from build123d import *

# Parameters (mm, degrees)
BOSS_EXTRUDE1_DEPTH      = 40
BOSS_EXTRUDE2_DEPTH      = 10
BOSS_EXTRUDE2_DEPTH_BACK = 50
SKETCH3_R                = 55


with BuildPart() as part:
    # Sketch2 → Boss-Extrude1 (new body)
    with BuildSketch(Plane(origin=(0, 0, 0), x_dir=(1, 0, 0), z_dir=(0, 1, 0))):
        Polygon((-545, 0), (545, 0), (614.776428685, 27.5), (614.776428685, -82.5), (545, -55), (-545, -55), (-614.776428685, -82.5), (-614.776428685, 27.5), align=None)
    extrude(amount=BOSS_EXTRUDE1_DEPTH)

    # Sketch3 → Boss-Extrude2 (add, two sides: drawn at the far end of the back side and taken through both)
    with BuildSketch(Plane(origin=(0, 40, 0), x_dir=(1, 0, 0), z_dir=(0, 1, 0)).offset(-BOSS_EXTRUDE2_DEPTH_BACK)):
        with Locations(Location((-614.776428685, -27.5, 0), (0, 0, 270))):
            Circle(SKETCH3_R)
        with Locations(Location((614.776428685, -27.5, 0), (0, 0, 270))):
            Circle(SKETCH3_R)
    extrude(amount=BOSS_EXTRUDE2_DEPTH + BOSS_EXTRUDE2_DEPTH_BACK)


solid = part.part
Input: part model. Units: mm. Frame: model coordinates. A direction names the side the tool comes from. Coordinates: 2 decimals unless noted, no trailing zeros. Loops run counter-clockwise (first coordinate to the right, second up) from the corner with the lowest first, then second, coordinate; pieces in that order, holes last.
(1) Section B-B on y = 17.5. Return the cut outline in (x, z).
(2) Section A-A on z = 27.5. Return the cut outline in (x, y).
(3) Material intervals for probe 1 along Y at (x, z) = (248.5, 14); probe 2 along Z at (x, y) = (-511, 22.5); probe 3 along X at (y, z) = (-1.5, -23), sorted ascending.
(4) First-contact query: pin 1 Ø1.5 at (x, z) = (-123.5, 18.5) entering from -Y; pin 2 Ø12 at (x, y) = (-278.5, 36.5) entering from -Z; pin 3 Ø1.5 at (y, z) = (13.5, 68) entering from -X. Flat tips, straight axial feed; report the tip coordinate or a pass-through.
(5) Section C-C on x = -224. Return the cut outline in (y, z).
(6) Pull-direction query (X, two-part tool) for faces 1 (the face through (669.31, 19.58, 20.34)), 2 (the face through (616, 50, 27)), 3 (the face through (-561.352, 19.72, -6.445)); classes: released by +X, released by -X, zero draft, split by the parting line, or undercut.
(7) Set-up query: faces 4 (the face through (-8, 20, 0)), 5 (the face through (-614, 50, 27)), 6 (the face through (-560.9, 19.72, 61.267)). Return all of +Z, -Z, +X, -X, +Y, -Y with unobstructed straight access to the full face (end or side cutting, diameter ignored); none if empty.
Data:
1. outline: (-577.25, -12.71) - (-545, 0) - (545, 0) - (577.25, -12.71) arc R55 ccw (long way) to (577.25, 67.71) - (545, 55) - (-545, 55) - (-577.25, 67.71) arc R55 ccw (long way) to start
2. outline: (-669.78, -10) - (-559.78, -10) - (-559.78, 0) - (559.78, 0) - (559.78, -10) - (669.78, -10) - (669.78, 50) - (559.78, 50) - (559.78, 40) - (-559.78, 40) - (-559.78, 50) - (-669.78, 50) - close
3. probe 1: y = 0 to 40
3. probe 2: z = 0 to 55
3. probe 3: x = -636.57 to -592.99, 592.99 to 636.57
4. pin 1: stops at y = 0
4. pin 2: stops at z = 0
4. pin 3: stops at x = -652.79
5. outline: (0, 0) - (40, 0) - (40, 55) - (0, 55) - close
6. face 1: undercut
6. face 2: zero draft
6. face 3: undercut
7. face 4: -Z, +Y, -Y
7. face 5: +Z, -Z, +X, -X, +Y
7. face 6: +Z, +Y, -Y
